Geometry check sheet. Reference: the model listing, model coordinates, mm. A direction names the side the tool comes from. Give positions to 0.01 mm unless a question says otherwise; leave off trailing zeros. Write each loop counter-clockwise with the first axis right and the second up, starting at its lowest first coordinate (ties: lowest second). Pieces come first, ordered by that corner, then holes. Notation, with made-up numbers: M -15.5,64.25 L -3.5,64.25 A20 ccw -3.5,93.25 Z; hole C 10.25,33.5 d8. An arc over 180 degrees is marked long. Write each question's results on one line, items separated by ' | '.
```python
from build123d import *

# Parameters (mm, degrees)
SKIZZE1_W                       = 44
SKIZZE1_H                       = 84.75
SKIZZE1_R                       = 9.125
SKIZZE1_R_2                     = 8.753791834
SKIZZE1_W_2                     = 18.25
SKIZZE1_H_2                     = 18.25
AUFSATZ_LINEAR_AUSTRAGEN1_DEPTH = 25
SKIZZE2_W                       = 7
SKIZZE2_H                       = 6.973629197
SKIZZE2_R                       = 1.8
AUFSATZ_LINEAR_AUSTRAGEN2_DEPTH = 2.5
SPIEGELN2_COPY_1_SKETCH_W       = 7
SPIEGELN2_COPY_1_SKETCH_H       = 6.973629197
SPIEGELN2_COPY_1_SKETCH_R       = 1.8
SPIEGELN2_COPY_1_DEPTH          = 2.5


with BuildPart() as part:
    # Skizze1 → Aufsatz-Linear austragen1 (new body)
    with BuildSketch(Plane(origin=(0, 0, 0), x_dir=(1, 0, 0), z_dir=(0, 1, 0))):
        Rectangle(SKIZZE1_W, SKIZZE1_H)
        with Locations((-10.375, 10)):
            Circle(SKIZZE1_R, mode=Mode.SUBTRACT)
        with Locations((10.375, 10)):
            Circle(SKIZZE1_R_2, mode=Mode.SUBTRACT)
        with Locations((-10.375, 30.75)):
            Rectangle(SKIZZE1_W_2, SKIZZE1_H_2, mode=Mode.SUBTRACT)
        with Locations((10.375, 30.75)):
            Rectangle(SKIZZE1_W_2, SKIZZE1_H_2, mode=Mode.SUBTRACT)
        with BuildLine():
            Line((-1.25, -10.75), (-1.25, -30.75))
            ThreePointArc((-1.25, -30.75), (-10.375, -39.875), (-19.5, -30.75))
            Line((-19.5, -30.75), (-19.5, -10.75))
            ThreePointArc((-19.5, -10.75), (-10.375, -1.625), (-1.25, -10.75))
        make_face(mode=Mode.SUBTRACT)
        with BuildLine():
            Line((19.5, -10.75), (19.5, -30.75))
            ThreePointArc((19.5, -30.75), (10.375, -39.875), (1.25, -30.75))
            Line((1.25, -30.75), (1.25, -10.75))
            ThreePointArc((1.25, -10.75), (10.375, -1.625), (19.5, -10.75))
        make_face(mode=Mode.SUBTRACT)
    extrude(amount=AUFSATZ_LINEAR_AUSTRAGEN1_DEPTH)

    # Skizze2 → Aufsatz-Linear austragen2 (add)
    with BuildSketch(Plane.XZ):
        with Locations((-25.5, 38.888185401)):
            Rectangle(SKIZZE2_W, SKIZZE2_H)
        with Locations((-25.5, 38.888185402)):
            Circle(SKIZZE2_R, mode=Mode.SUBTRACT)
    aufsatz_linear_austragen2 = extrude(amount=-AUFSATZ_LINEAR_AUSTRAGEN2_DEPTH)

    # Spiegeln1: Aufsatz-Linear austragen2 across plane
    add(aufsatz_linear_austragen2.mirror(Plane(origin=(0, 0, 0), x_dir=(0, 0, 1), z_dir=(1, 0, 0))))

    # Spiegeln2: Aufsatz-Linear austragen2 across plane
    add(aufsatz_linear_austragen2.mirror(Plane.XY))

    # Spiegeln2 copy 1 sketch → Spiegeln2 copy 1 (add)
    with BuildSketch(Plane(origin=(0, 0, 0), x_dir=(-1, 0, 0), z_dir=(0, -1, 0))):
        with Locations((-25.5, 38.888185401)):
            Rectangle(SPIEGELN2_COPY_1_SKETCH_W, SPIEGELN2_COPY_1_SKETCH_H)
        with Locations((-25.5, 38.888185402)):
            Circle(SPIEGELN2_COPY_1_SKETCH_R, mode=Mode.SUBTRACT)
    extrude(amount=-SPIEGELN2_COPY_1_DEPTH)


solid = part.part
```
Q1. Access from +Z, -Z, +X, -X, +Y, -Y to the whole of each face (thin tool, end or side, straight path). Record for faces 1 (the face through (10.174, 12.325, 1.627)), 2 (the face through (26, 1, -35.401)), 3 (the face through (-27.1, 2.5, -40.5)), 4 (the face through (27.1, 2.5, -40.5)), 5 (the face through (-26, 1, -35.401)).
Answer key:
face 1: +Y, -Y | face 2: +X, +Y, -Y | face 3: +Z, -Z, -X, +Y | face 4: +Z, -Z, +X, +Y | face 5: -X, +Y, -Y
Q2. Section check B-B (y = 16.75). Enter the section's corners in (x, z) (3 decimals), then the cut area to 3 significant figures.
Answer key:
outline: M -22,-42.375 L 22,-42.375 L 22,42.375 L -22,42.375 Z; hole M -19.5,-39.875 L -1.25,-39.875 L -1.25,-21.625 L -19.5,-21.625 Z; hole C -10.375,-10 d18.25; hole M -19.5,10.75 A9.125 ccw -1.25,10.75 L -1.25,30.75 A9.125 ccw -19.5,30.75 Z; hole M 1.25,-39.875 L 19.5,-39.875 L 19.5,-21.625 L 1.25,-21.625 Z; hole M 1.25,10.75 A9.125 ccw 19.5,10.75 L 19.5,30.75 A9.125 ccw 1.25,30.75 Z; hole C 10.375,-10 d17.508 | area: 1,310 mm2
Q3. Section check C-C (x = -25.5). Enter the section's corners in (y, z) (3 decimals), then the cut area to 3 significant figures.
Answer key:
outline: M 0,-42.375 L 2.5,-42.375 L 2.5,-40.688 L 0,-40.688 Z; M 0,-37.088 L 2.5,-37.088 L 2.5,-35.401 L 0,-35.401 Z; M 0,35.401 L 2.5,35.401 L 2.5,37.088 L 0,37.088 Z; M 0,40.688 L 2.5,40.688 L 2.5,42.375 L 0,42.375 Z | area: 16.9 mm2
Q4. Material ranges on probe 1 along X at (y, z) = (10.75, -35.5); probe 2 along X at (y, z) = (16.25, -9.5); probe 3 along Z at (x, y) = (25.5, 1.95) (3 decimals), recorded low to high. Write a range as [from, to].
Answer key:
probe 1: x = [-22, -19.5], [-1.25, 1.25], [19.5, 22] | probe 2: x = [-22, -19.49], [-1.26, 1.64], [19.11, 22] | probe 3: z = [-42.375, -40.688], [-37.088, -35.401], [35.401, 37.088], [40.688, 42.375]
Q5. Section check A-A (z = -24.5). Enter the section's corners in (x, y), then the cut area to 4 significant figures.
Answer key:
outline: M -22,0 L -19.5,0 L -19.5,25 L -22,25 Z; M -1.25,0 L 1.25,0 L 1.25,25 L -1.25,25 Z; M 19.5,0 L 22,0 L 22,25 L 19.5,25 Z | area: 187.5 mm2
Q6. Depth check by flat-ended pin: P1, Ø7.5, axis at y = 12.5, z = -2, coming from the +X side; P2, Ø14.5, axis at y = 15.5, z = -30.5, coming from the -X side; P3, Ø4.5, axis at x = -25.5, z = 38.89, coming from the +Y side; P4, Ø1.5, axis at x = -21.5, z = 11.5, coming from the -Y side. Enter the tip coordinate at first touch or a pass-through.
Answer key:
P1: stops at x = 22 | P2: stops at x = -22 | P3: stops at y = 2.5 | P4: stops at y = 0
Q7. Release check for a two-part mould opening along Z. For faces 6 (the face through (-29, 1, -39)), 7 (the face through (-11, 12, -21.625)) record: released by +Z, released by -Z, zero draft, split by the parting line, or undercut.
Answer key:
face 6: zero draft | face 7: undercut
Q8. Section check D-D (z = -10). Enter the section's corners in (x, y).
Answer key:
outline: M -22,0 L -19.5,0 L -19.5,25 L -22,25 Z; M -1.25,0 L 1.62,0 L 1.62,25 L -1.25,25 Z; M 19.13,0 L 22,0 L 22,25 L 19.13,25 Z
